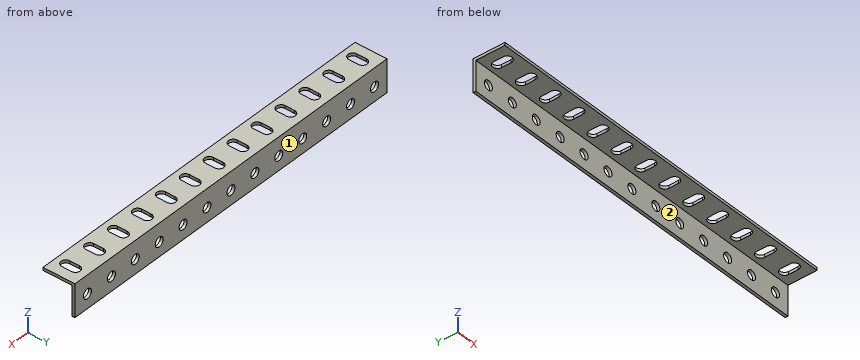
```python
from build123d import *

# Parameters (mm, degrees)
SKETCH1_W           = 165.42
SKETCH1_H           = 14.34
BOSS_EXTRUDE1_DEPTH = 1.3
SKETCH3_W           = 165.42
SKETCH3_H           = 14.62
SKETCH3_R           = 2.11
BOSS_EXTRUDE2_DEPTH = 1.3


with BuildPart() as part:
    # Sketch1 → Boss-Extrude1 (new body)
    with BuildSketch(Plane.XY):
        with Locations((0, 0.39)):
            Rectangle(SKETCH1_W, SKETCH1_H)
        with BuildLine():
            Line((-73.97, 2.15), (-73.97, -2.15))
            ThreePointArc((-73.97, -2.15), (-76.08, -4.26), (-78.19, -2.15))
            Line((-78.19, -2.15), (-78.19, 2.15))
            ThreePointArc((-78.19, 2.15), (-76.08, 4.26), (-73.97, 2.15))
        make_face(mode=Mode.SUBTRACT)
        with BuildLine():
            Line((-65.51, 2.15), (-65.51, -2.15))
            ThreePointArc((-65.51, -2.15), (-63.4, -4.26), (-61.29, -2.15))
            Line((-61.29, -2.15), (-61.29, 2.15))
            ThreePointArc((-61.29, 2.15), (-63.4, 4.26), (-65.51, 2.15))
        make_face(mode=Mode.SUBTRACT)
        with BuildLine():
            Line((-52.83, 2.15), (-52.83, -2.15))
            ThreePointArc((-52.83, -2.15), (-50.72, -4.26), (-48.61, -2.15))
            Line((-48.61, -2.15), (-48.61, 2.15))
            ThreePointArc((-48.61, 2.15), (-50.72, 4.26), (-52.83, 2.15))
        make_face(mode=Mode.SUBTRACT)
        with BuildLine():
            Line((-40.15, 2.15), (-40.15, -2.15))
            ThreePointArc((-40.15, -2.15), (-38.04, -4.26), (-35.93, -2.15))
            Line((-35.93, -2.15), (-35.93, 2.15))
            ThreePointArc((-35.93, 2.15), (-38.04, 4.26), (-40.15, 2.15))
        make_face(mode=Mode.SUBTRACT)
        with BuildLine():
            Line((-27.47, 2.15), (-27.47, -2.15))
            ThreePointArc((-27.47, -2.15), (-25.36, -4.26), (-23.25, -2.15))
            Line((-23.25, -2.15), (-23.25, 2.15))
            ThreePointArc((-23.25, 2.15), (-25.36, 4.26), (-27.47, 2.15))
        make_face(mode=Mode.SUBTRACT)
        with BuildLine():
            Line((-14.79, 2.15), (-14.79, -2.15))
            ThreePointArc((-14.79, -2.15), (-12.68, -4.26), (-10.57, -2.15))
            Line((-10.57, -2.15), (-10.57, 2.15))
            ThreePointArc((-10.57, 2.15), (-12.68, 4.26), (-14.79, 2.15))
        make_face(mode=Mode.SUBTRACT)
        with BuildLine():
            Line((-2.11, 2.15), (-2.11, -2.15))
            ThreePointArc((-2.11, -2.15), (0, -4.26), (2.11, -2.15))
            Line((2.11, -2.15), (2.11, 2.15))
            ThreePointArc((2.11, 2.15), (0, 4.26), (-2.11, 2.15))
        make_face(mode=Mode.SUBTRACT)
        with BuildLine():
            Line((10.57, 2.15), (10.57, -2.15))
            ThreePointArc((10.57, -2.15), (12.68, -4.26), (14.79, -2.15))
            Line((14.79, -2.15), (14.79, 2.15))
            ThreePointArc((14.79, 2.15), (12.68, 4.26), (10.57, 2.15))
        make_face(mode=Mode.SUBTRACT)
        with BuildLine():
            Line((23.25, 2.15), (23.25, -2.15))
            ThreePointArc((23.25, -2.15), (25.36, -4.26), (27.47, -2.15))
            Line((27.47, -2.15), (27.47, 2.15))
            ThreePointArc((27.47, 2.15), (25.36, 4.26), (23.25, 2.15))
        make_face(mode=Mode.SUBTRACT)
        with BuildLine():
            Line((35.93, 2.15), (35.93, -2.15))
            ThreePointArc((35.93, -2.15), (38.04, -4.26), (40.15, -2.15))
            Line((40.15, -2.15), (40.15, 2.15))
            ThreePointArc((40.15, 2.15), (38.04, 4.26), (35.93, 2.15))
        make_face(mode=Mode.SUBTRACT)
        with BuildLine():
            Line((48.61, 2.15), (48.61, -2.15))
            ThreePointArc((48.61, -2.15), (50.72, -4.26), (52.83, -2.15))
            Line((52.83, -2.15), (52.83, 2.15))
            ThreePointArc((52.83, 2.15), (50.72, 4.26), (48.61, 2.15))
        make_face(mode=Mode.SUBTRACT)
        with BuildLine():
            Line((61.29, 2.15), (61.29, -2.15))
            ThreePointArc((61.29, -2.15), (63.4, -4.26), (65.51, -2.15))
            Line((65.51, -2.15), (65.51, 2.15))
            ThreePointArc((65.51, 2.15), (63.4, 4.26), (61.29, 2.15))
        make_face(mode=Mode.SUBTRACT)
        with BuildLine():
            Line((73.97, 2.15), (73.97, -2.15))
            ThreePointArc((73.97, -2.15), (76.08, -4.26), (78.19, -2.15))
            Line((78.19, -2.15), (78.19, 2.15))
            ThreePointArc((78.19, 2.15), (76.08, 4.26), (73.97, 2.15))
        make_face(mode=Mode.SUBTRACT)
    extrude(amount=-BOSS_EXTRUDE1_DEPTH)

    # Sketch3 → Boss-Extrude2 (add)
    with BuildSketch(Plane(origin=(0, 7.56, 0), x_dir=(1, 0, 0), z_dir=(0, 1, 0))):
        with Locations((0, 7.31)):
            Rectangle(SKETCH3_W, SKETCH3_H)
        with Locations(Location((-76.08, 8.19, 0), (0, 0, 270))):
            Circle(SKETCH3_R, mode=Mode.SUBTRACT)
        with Locations(Location((-63.4, 8.19, 0), (0, 0, 270))):
            Circle(SKETCH3_R, mode=Mode.SUBTRACT)
        with Locations(Location((-50.72, 8.19, 0), (0, 0, 270))):
            Circle(SKETCH3_R, mode=Mode.SUBTRACT)
        with Locations(Location((-38.04, 8.19, 0), (0, 0, 270))):
            Circle(SKETCH3_R, mode=Mode.SUBTRACT)
        with Locations(Location((-25.36, 8.19, 0), (0, 0, 270))):
            Circle(SKETCH3_R, mode=Mode.SUBTRACT)
        with Locations(Location((-12.68, 8.19, 0), (0, 0, 270))):
            Circle(SKETCH3_R, mode=Mode.SUBTRACT)
        with Locations(Location((0, 8.19, 0), (0, 0, 270))):
            Circle(SKETCH3_R, mode=Mode.SUBTRACT)
        with Locations(Location((12.68, 8.19, 0), (0, 0, 270))):
            Circle(SKETCH3_R, mode=Mode.SUBTRACT)
        with Locations(Location((25.36, 8.19, 0), (0, 0, 270))):
            Circle(SKETCH3_R, mode=Mode.SUBTRACT)
        with Locations(Location((38.04, 8.19, 0), (0, 0, 270))):
            Circle(SKETCH3_R, mode=Mode.SUBTRACT)
        with Locations(Location((50.72, 8.19, 0), (0, 0, 270))):
            Circle(SKETCH3_R, mode=Mode.SUBTRACT)
        with Locations(Location((63.4, 8.19, 0), (0, 0, 270))):
            Circle(SKETCH3_R, mode=Mode.SUBTRACT)
        with Locations(Location((76.08, 8.19, 0), (0, 0, 270))):
            Circle(SKETCH3_R, mode=Mode.SUBTRACT)
    extrude(amount=-BOSS_EXTRUDE2_DEPTH)


solid = part.part
```
Part model, mm, in its own coordinate system. Face numbers are marked on the shaded views. A direction names the side the tool comes from. Round coordinates to 2 decimals unless told otherwise and drop trailing zeros. Loops run counter-clockwise (first coordinate to the right, second up) from the corner with the lowest first, then second, coordinate; pieces in that order, holes last. Notation, with made-up numbers: (42.5, 55.25) -> (67.5, 55.25) arc R18 cw to (67.5, 75.25) -> close; hole circle Ø7 at (39, 45). An arc over 180 degrees is marked (long way). Use one line per item in the form item = value. Start each with the question number.
Item 1: Band-saw the part on B-B (x = -5.5). List the corners of the cut face in (y, z), plus the area to 3 significant figures.
Item 2: Drill centre lines: line 1 along Z through (x, y) = (-32, 4.75); line 2 along Y through (x, z) = (60, -12.5). Where is each one in solid material? Low to high.
Item 3: Tool access for the marked faces 1 and 2: list every direction of +Z, -Z, +X, -X, +Y, -Y with a clear straight run to the whole face (end or side of a thin tool).
Item 4: Drop flat-ended pins along their axis: pin 1 Ø5 at (x, z) = (63.4, -8.19) entering from -Y; pin 2 Ø1 at (x, y) = (31, 0.5) entering from -Z; pin 3 Ø2.5 at (x, z) = (76.08, -8.19) entering from +Y. Give the stop position or say it passes through.
Item 5: Band-saw the part on A-A (x = 38.04). List the corners of the cut face in (y, z), plus the area to 3 significant figures.
Item 6: Band-saw the part on C-C (z = -2.75). List the corners of the cut face in (x, y), plus the area to 3 significant figures.
Data:
q1.outline = (-6.78, -1.3) -> (6.26, -1.3) -> (6.26, -14.62) -> (7.56, -14.62) -> (7.56, 0) -> (-6.78, 0) -> close
q1.area = 36.0 mm^2
q2.line_1 = -1.3 to 0
q2.line_2 = 6.26 to 7.56
q3.face_1 = +Z, -Z, +X, -X, +Y
q3.face_2 = -Z, +X, -X, -Y
q4.pin_1 = 6.26
q4.pin_2 = -1.3
q4.pin_3 = through
q5.outline = (-6.78, -1.3) -> (-4.26, -1.3) -> (-4.26, 0) -> (-6.78, 0) -> close; (4.26, -1.3) -> (6.26, -1.3) -> (6.26, -6.08) -> (7.56, -6.08) -> (7.56, 0) -> (4.26, 0) -> close; (6.26, -14.62) -> (7.56, -14.62) -> (7.56, -10.3) -> (6.26, -10.3) -> close
q5.area = 19.4 mm^2
q6.outline = (-82.71, 6.26) -> (82.71, 6.26) -> (82.71, 7.56) -> (-82.71, 7.56) -> close
q6.area = 215 mm^2
